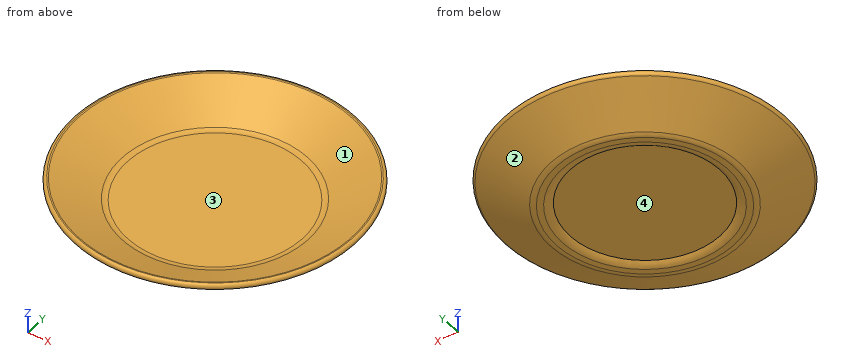
```python
from build123d import *

# Parameters (mm, degrees)
F0_R     = 38.8061370384
F2_R     = 63.433920718
F4_T     = -2.54
F5_R     = 1.26999
F6_R     = 31.6978703438
F7_DEPTH = 1.27
F9_R     = 5.08


# Not quite as in the source:
# - a fillet or chamfer that OpenCascade refuses, or shapes differently, is made with other operations: its cross-section is extruded or revolved along the edge and cut away or added
# - a fillet or chamfer is up to 0.001 mm smaller than in the source, because OpenCascade refuses the exact size


with BuildPart() as f3:
    # F0 (on Top) → F3 section 0
    with BuildSketch(Plane.XY):
        Circle(F0_R)
    # F2 (on offset) → F3 section 1
    with BuildSketch(Plane.XY.offset(12.7)):
        Circle(F2_R)
    loft()

    # F4
    f4_openings = [f3.faces().sort_by_distance(p)[0] for p in [
        (0, 0, 12.7),
    ]]
    offset(amount=F4_T, openings=f4_openings, kind=Kind.INTERSECTION)

    # F5 (radius 1.27 in the source; OpenCascade refuses exactly that, so slightly less here)
    f5_edges = [f3.edges().sort_by_distance(p)[0] for p in [
        (-63.433921, 0, 12.7),
        (-57.892016, 0, 12.7),
    ]]
    fillet(f5_edges, radius=F5_R)

    # F6 (on face) → F7 (cut)
    with BuildSketch(Plane(origin=(0, 0, 0), x_dir=(1, 0, 0), z_dir=(0, 0, -1))):
        Circle(F6_R)
    extrude(amount=-F7_DEPTH, mode=Mode.SUBTRACT)

    # F8: fillet of radius 5.08 on 2 edges, made by hand

    # F8_s1 → F8_t2 (revolve, cut)
    with BuildSketch(Plane.XZ):
        with BuildLine():
            ThreePointArc((35.0579745088, 0), (33.2619232846, 0.3280951188), (31.6978703438, 1.27))
            Line((31.6978703438, 1.27), (31.6978703438, 0))
            Line((31.6978703438, 0), (35.0579745088, 0))
        make_face()
    revolve(axis=Axis((0, 0, 0), (0, 0, -1)), mode=Mode.SUBTRACT)

    # F8_s3 → F8_t4 (revolve, cut)
    with BuildSketch(Plane.XZ):
        with BuildLine():
            ThreePointArc((39.9017377768, 0.5649769203), (38.7713729734, 0.1432643759), (37.5734408477, 0))
            Line((37.5734408477, 0), (38.8061370384, 0))
            Line((38.8061370384, 0), (39.9017377768, 0.5649769203))
        make_face()
    revolve(axis=Axis((0, 0, 0), (0, 0, 1)), mode=Mode.SUBTRACT)

    # F9
    f9_edges = [f3.edges().sort_by_distance(p)[0] for p in [
        (-38.189789, 0, 2.54),
    ]]
    fillet(f9_edges, radius=F9_R)


solid = f3.part
```
The listing builds one solid part. Answer for the finished solid, in the listing's coordinates (mm). Face numbers are marked on the shaded views. A direction names the side the tool comes from. Give positions to 0.01 mm unless a question says otherwise; leave off trailing zeros. Answer as a JSON object with one key per item and string values. Group by question number.
Item 1: Determine the mould class of the marked faces 1 and 2 for opening direction X: pulls with the +X half, pulls with the -X half, needs draft (parallel to the pull), parting line crosses it, or undercut.
Item 2: A tool of negligible diameter and unlimited length cuts with its end or side. For the marked faces 3 and 4, from which of +Z, -Z, +X, -X, +Y, -Y can it reach the whole face along a straight path? Write none if from no direction.
Item 3: Consider L1, parallel to Z at x = -27.5, y = -9; L2, parallel to X at y = -1.5, z = 3.5; L3, parallel to Y at x = 30, z = 7.5. Determine where each line is inside the solid, lowest interval first. Write a range as from..to.
Item 4: Flat-ended cylindrical pins translate along their axes: pin 1 (3 mm diameter, centred on x = 11.5, y = -14.5, fed in from -Z); pin 2 (4 mm diameter, centred on y = 44.5, z = 9, fed in from -X); pin 3 (1 mm diameter, centred on x = -16.5, z = 1.5, fed in from +Y). Find the tip coordinate at first contact, or state that the pin passes through.
Result set:
{
 "1": {"face 1": "undercut", "face 2": "parting line crosses it"},
 "2": {"face 3": "+Z", "face 4": "-Z"},
 "3": {"L1": "1.27..2.54", "L2": "-45.57..-40.02, 40.02..45.57", "L3": "-44.12..-37.22, 37.22..44.12"},
 "4": {"pin 1": "z = 1.27", "pin 2": "x = -40.32", "pin 3": "y = 39.39"}
}
